Answer from the drawing. Dimensions are ordinates in mm from the lowest x, y and z of the part. A direction names the side the tool comes from. Give positions to 0.01 mm unless a question says otherwise; leave off trailing zeros. Order: outer loops, then holes, each group sorted by start corner. A loop starts at its lowest first (then second) coordinate and runs counter-clockwise, first axis right, second up.
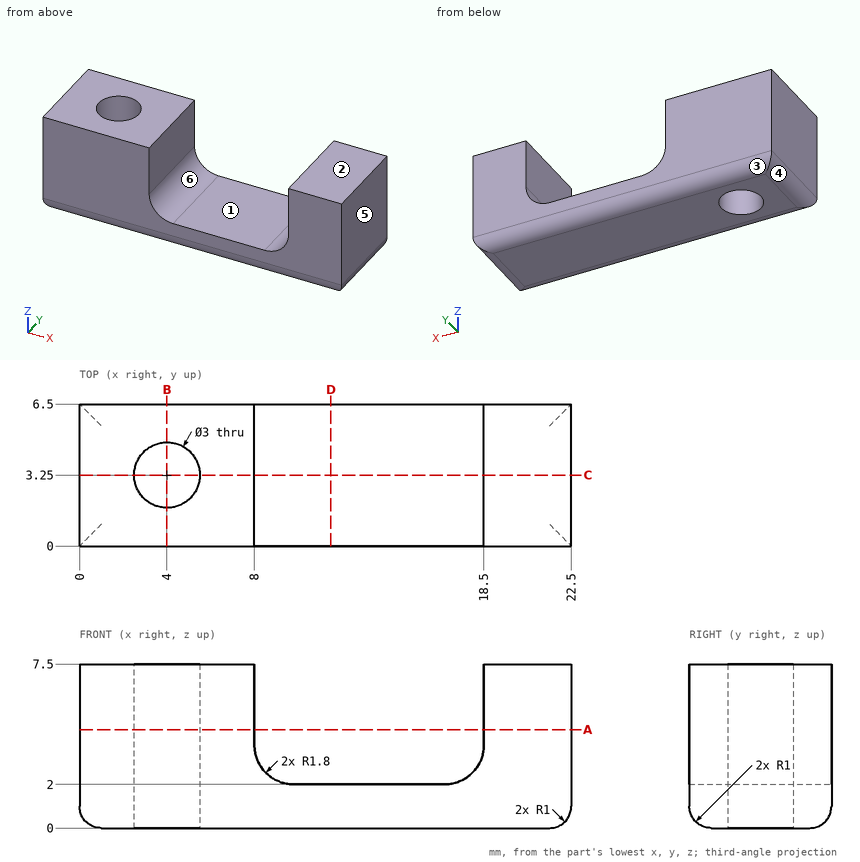
1. The part is cut by section B-B (x = 4). Write down the section's boundary in (y, z).
Findings below:
outline: (0, 1) arc R1 ccw to (1, 0) - (1.75, 0) - (1.75, 7.5) - (0, 7.5) - close; (4.75, 0) - (5.5, 0) arc R1 ccw to (6.5, 1) - (6.5, 7.5) - (4.75, 7.5) - close
2. Straight lines are drawn through the part: probe 1 along Y at (x, z) = (4, 3.25); probe 2 along X at (y, z) = (4.25, 5.25); probe 3 along X at (y, z) = (4.5, 7.25). For each, find the intervals that lie inside material, in ascending order.
Findings below:
probe 1: y = 0 to 1.75, 4.75 to 6.5
probe 2: x = 0 to 2.88, 5.12 to 8, 18.5 to 22.5
probe 3: x = 0 to 3.17, 4.83 to 8, 18.5 to 22.5
3. The mould has two halves that part along X. Classify the marked faces 3, 4, 5 and 6: pulls with the +X half, pulls with the -X half, needs draft (parallel to the pull), parting line crosses it, or undercut.
Findings below:
face 3: needs draft
face 4: pulls with the -X half
face 5: pulls with the +X half
face 6: undercut
4. The part is cut by section D-D (x = 11.5). Write down the section's boundary in (y, z).
Findings below:
outline: (0, 1) arc R1 ccw to (1, 0) - (5.5, 0) arc R1 ccw to (6.5, 1) - (6.5, 2) - (0, 2) - close
5. Given P1, Ø1.5, axis at x = 10.5, y = 2, coming from the -Z side, flat-ended and moving along its own axis, determine where the tip first touches the part or whether it passes through.
Findings below:
P1: stops at z = 0
6. The part is cut by section C-C (y = 3.25). Write down the section's boundary in (x, z).
Findings below:
outline: (0, 1) arc R1 ccw to (1, 0) - (2.5, 0) - (2.5, 7.5) - (0, 7.5) - close; (5.5, 0) - (21.5, 0) arc R1 ccw to (22.5, 1) - (22.5, 7.5) - (18.5, 7.5) - (18.5, 3.8) arc R1.8 cw to (16.7, 2) - (9.8, 2) arc R1.8 cw to (8, 3.8) - (8, 7.5) - (5.5, 7.5) - close
7. The part is cut by section A-A (z = 4.5). Write down the section's boundary in (x, y).
Findings below:
outline: (0, 0) - (8, 0) - (8, 6.5) - (0, 6.5) - close; (18.5, 0) - (22.5, 0) - (22.5, 6.5) - (18.5, 6.5) - close; hole circle Ø3 at (4, 3.25)
8. Which of the six approach directions +Z, -Z, +X, -X, +Y, -Y give full straight-line access (tool end or side, diameter ignored) to the marked faces 1 and 2?
Findings below:
face 1: +Z, +Y, -Y
face 2: +Z, +X, -X, +Y, -Y
